Study the drawing (mm; zero at the part's minimum x, y, z) and answer. A direction names the side the tool comes from. Round coordinates to 2 decimals unless told otherwise and drop trailing zeros. Write each loop counter-clockwise with the first axis right and the second up, starting at its lowest first coordinate (ties: lowest second). Pieces come first, ordered by that corner, then holes. Notation, with made-up numbers: (16.5, 73.25) - (39.5, 73.25) arc R18 cw to (39.5, 101.25) - close; hole circle Ø4 at (80, 33). An arc over 180 degrees is marked (long way). Return JSON: item names as keys, results as strings. Group by question number.
(1) Find the intervals of material crossed by line 1 along X through (y, z) = (6.5, 1.5) (1 decimal); line 2 along Y through (x, z) = (2, 1.1); line 3 along Y through (x, z) = (3.5, 1.75), in increasing order. Write a range as [from, to].
(2) Section C-C, the plane y = 14 is taken. Write down the section's boundary in (x, z) (3 decimals).
(3) Each of these flat-tipped pins is pushed along its axis until it touches: pin 1 (1 mm diameter, centred on y = 8.5, z = 0.5, fed in from -X) (3 decimals); pin 2 (0.8 mm diameter, centred on y = 14, z = 1.5, fed in from +X); pin 3 (1 mm diameter, centred on x = 4.5, z = 1, fed in from -Y). Where does it stop, or does it pass through?
(4) Which of the six approach directions +Z, -Z, +X, -X, +Y, -Y give full straight-line access (tool end or side, diameter ignored) to the marked faces 5, 6 and 7?
(5) Section D-D, the plane y = 10 is taken. Write down the section's boundary in (x, z) (3 decimals), then the cut area to 3 significant figures.
(6) Section B-B, the plane z = 0.95 is taken. Write down the section's boundary in (x, y) (3 decimals).
(7) Determine the mould class of the marked faces 1, 2, 3 and 4 for opening direction X: +X half, -X half, draft (parallel to the pull), parting line (faces both ways), or undercut.
(8) Section A-A, the plane x = 5.75 is taken. Write down the section's boundary in (y, z).
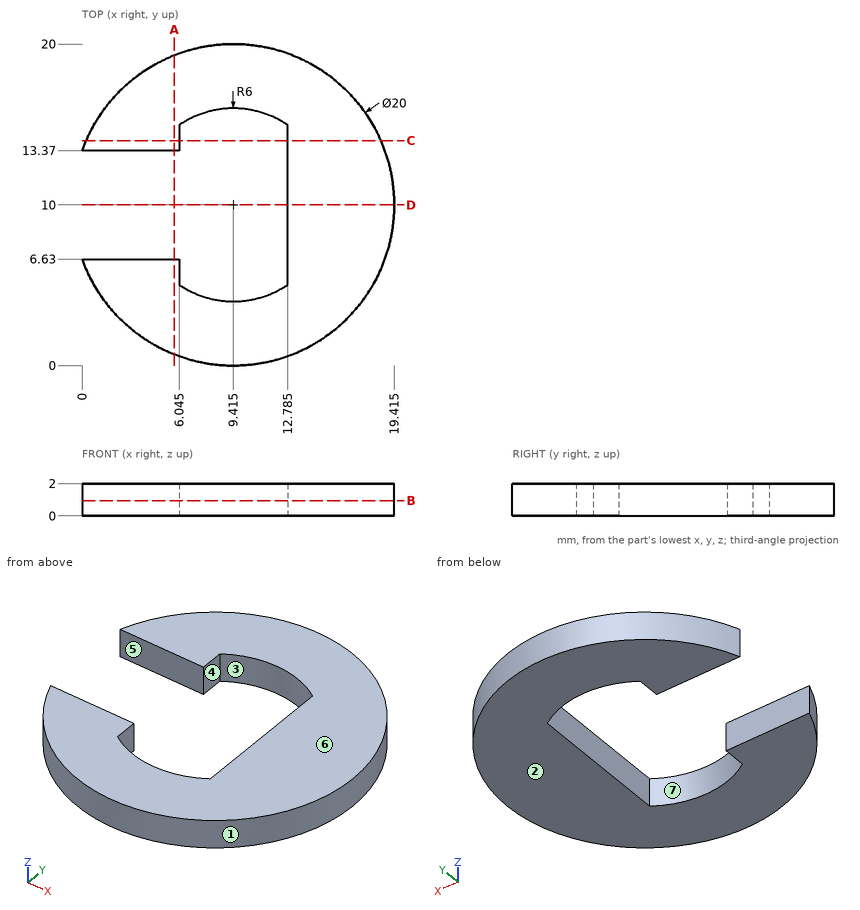
Working result:
{
 "1": {"line 1": "x = [0, 6], [12.8, 18.8]", "line 2": "y = [3.29, 6.63], [13.37, 16.71]", "line 3": "y = [1.94, 6.63], [13.37, 18.06]"},
 "2": {"outline": "(0.25, 0) - (6.045, 0) - (6.045, 2) - (0.25, 2) - close; (12.785, 0) - (18.58, 0) - (18.58, 2) - (12.785, 2) - close"},
 "3": {"pin 1": "stops at x = 12.785", "pin 2": "stops at x = 18.74", "pin 3": "stops at y = 1.03"},
 "4": {"face 5": "+Z, -Z, -X", "face 6": "+Z, +X, -X, +Y, -Y", "face 7": "+Z, -Z"},
 "5": {"outline": "(12.785, 0) - (19.415, 0) - (19.415, 2) - (12.785, 2) - close", "area": "13.3 mm^2"},
 "6": {"outline": "(0, 6.63) arc R10 ccw (long way) to (0, 13.37) - (6.045, 13.37) - (6.045, 14.964) arc R6 cw to (12.785, 14.964) - (12.785, 5.036) arc R6 cw to (6.045, 5.036) - (6.045, 6.63) - close"},
 "7": {"face 1": "parting line", "face 2": "draft", "face 3": "undercut", "face 4": "undercut"},
 "8": {"outline": "(0.7, 0) - (6.63, 0) - (6.63, 2) - (0.7, 2) - close; (13.37, 0) - (19.3, 0) - (19.3, 2) - (13.37, 2) - close"}
}
